```python
from build123d import *

# Parameters (mm, degrees)
SKETCH1_R           = 2.286
SKETCH1_R_2         = 1.905
SKETCH1_W           = 6.35
SKETCH1_H           = 6.35
BOSS_EXTRUDE1_DEPTH = 6.35
FILLET1_R           = 6.35


with BuildPart() as part:
    # Sketch1 → Boss-Extrude1 (new body)
    with BuildSketch(Plane.XY):
        with BuildLine():
            Line((0, 0), (-25.4, 0))
            Line((-25.4, 0), (-44.325080611, 93.996655919))
            ThreePointArc((-44.325080611, 93.996655919), (-40.259800646, 101.221411991), (-32.513467201, 98.268799644))
            Line((-32.513467201, 98.268799644), (0, 38.1))
            Line((0, 38.1), (15.393399204, 0))
            Line((15.393399204, 0), (0, 0))
        make_face()
        with Locations((-6.35, 6.35)):
            Circle(SKETCH1_R, mode=Mode.SUBTRACT)
        with Locations((-19.05, 31.75)):
            Circle(SKETCH1_R, mode=Mode.SUBTRACT)
        with Locations((-38.1, 86.995)):
            Circle(SKETCH1_R_2, mode=Mode.SUBTRACT)
        with Locations((-38.1, 95.25)):
            Rectangle(SKETCH1_W, SKETCH1_H, mode=Mode.SUBTRACT)
    extrude(amount=-BOSS_EXTRUDE1_DEPTH)

    # Fillet1
    fillet1_edges = [part.edges().sort_by_distance(p)[0] for p in [
        (15.393399204, 0, -3.175),
    ]]
    fillet(fillet1_edges, radius=FILLET1_R)


solid = part.part
```
Source: CAD feature listing. Evaluate the final solid. Frame: model axes, mm. A direction names the side the tool comes from. Give positions to 0.01 mm unless a question says otherwise; leave off trailing zeros. Order: outer loops, then holes, each group sorted by start corner. A loop starts at its lowest first (then second) coordinate and runs counter-clockwise, first axis right, second up. Notation, with made-up numbers: (-10.75, 37.5) -> (33.25, 37.5) arc R13 cw to (33.25, 57.5) -> close; hole circle Ø1 at (33, -9). An arc over 180 degrees is marked (long way). Use a Markdown table: item, result.
Q1. Material intervals for line 1 (Y direction, x = -19.05, z = -1.25); line 2 (Y direction, x = -6.35, z = -5); line 3 (X direction, y = 10, z = -2.5), sorted ascending. Write a range as [from, to].
A:
| item | result |
|---|---|
| line 1 | [0, 29.46], [34.04, 73.35] |
| line 2 | [0, 4.06], [8.64, 49.85] |
| line 3 | [-27.41, 11.35] |
Q2. Section A-A (x = -18). Return the cut outline in (y, z).
A:
| item | result |
|---|---|
| outline | (0, -6.35) -> (29.72, -6.35) -> (29.72, 0) -> (0, 0) -> close; (33.78, -6.35) -> (71.41, -6.35) -> (71.41, 0) -> (33.78, 0) -> close |
Q3. Section B-B (z = -3.25). Return the cut outline in (x, y) (3 decimals), and give its area (3 significant figures).
A:
| item | result |
|---|---|
| outline | (-44.325, 93.997) -> (-25.4, 0) -> (5.979, 0) arc R6.35 ccw to (11.867, 8.729) -> (0, 38.1) -> (-32.513, 98.269) arc R6.35 ccw to start; hole (-41.275, 92.075) -> (-34.925, 92.075) -> (-34.925, 98.425) -> (-41.275, 98.425) -> close; hole circle Ø3.81 at (-38.1, 86.995); hole circle Ø4.572 at (-19.05, 31.75); hole circle Ø4.572 at (-6.35, 6.35) |
| area | 2,700 mm^2 |
Q4. Section C-C (y = 31.75). Return the cut outline in (x, z), and give its area (3 significant figures).
A:
| item | result |
|---|---|
| outline | (-31.79, -6.35) -> (-21.34, -6.35) -> (-21.34, 0) -> (-31.79, 0) -> close; (-16.76, -6.35) -> (2.57, -6.35) -> (2.57, 0) -> (-16.76, 0) -> close |
| area | 189 mm^2 |
Q5. Pull-direction query (Y, two-part tool) for faces 1 (the face through (11.194, 2.727, -3.219)), 2 (the face through (-16, 40, -6.35)), 3 (the face through (-38.513, 85.135, -3.131)), 4 (the face through (-9, 0, -3)); classes: +Y half, -Y half, draft (parallel to the pull), parting line (faces both ways), or undercut.
A:
| item | result |
|---|---|
| face 1 | parting line |
| face 2 | draft |
| face 3 | undercut |
| face 4 | -Y half |
Q6. First-contact query: P1, Ø3, axis at y = 95.5, z = -4.5, coming from the +X side. Flat tip, straight axial feed; report the tip coordinate or a pass-through.
A:
| item | result |
|---|---|
| P1 | x = -30.21 |
Q7. Section D-D (x = -38.1). Return the cut outline in (y, z) (3 decimals).
A:
| item | result |
|---|---|
| outline | (63.078, -6.35) -> (85.09, -6.35) -> (85.09, 0) -> (63.078, 0) -> close; (88.9, -6.35) -> (92.075, -6.35) -> (92.075, 0) -> (88.9, 0) -> close; (98.425, -6.35) -> (101.6, -6.35) -> (101.6, 0) -> (98.425, 0) -> close |
Q8. Access query for faces 5 (the face through (5.85, 23.62, -3.13)), 6 (the face through (-38, 92.075, -3)). Directions: +Z, -Z, +X, -X, +Y, -Y. A direction counts if a zero-diameter tool reaches every point of the face in a straight line with its end or side. Return the directions, or none.
A:
| item | result |
|---|---|
| face 5 | +Z, -Z, +X, +Y |
| face 6 | +Z, -Z |
